from build123d import *

# Parameters (mm, degrees)
F1_DEPTH = 60
F2_R     = 5
F3_SIZE  = 5
F4_R     = 22.693936
F5_DEPTH = 30


with BuildPart() as f1:
    # F0 (on Front) → F1 (new body)
    with BuildSketch(Plane.XZ):
        with BuildLine():
            Line((58.700657, 72.187497), (-16.299343, 72.187497))
            ThreePointArc((-16.299343, 72.187497), (-33.977013, 64.865167), (-41.299343, 47.187497))
            Line((-41.299343, 47.187497), (-41.299343, -27.812503))
            Line((-41.299343, -27.812503), (33.700657, -27.812503))
            ThreePointArc((33.700657, -27.812503), (51.378326, -20.490172), (58.700657, -2.812503))
            Line((58.700657, -2.812503), (58.700657, 72.187497))
        make_face()
    extrude(amount=F1_DEPTH)

    # F2
    f2_edges = [f1.edges().sort_by_distance(p)[0] for p in [
        (58.700657, -60, 34.687497),
        (21.200657, -60, 72.187497),
        (-33.977013, -60, 64.865167),
        (-41.299343, -60, 9.687497),
        (-3.799343, -60, -27.812503),
        (51.378326, -60, -20.490172),
    ]]
    fillet(f2_edges, radius=F2_R)

    # F3
    f3_edges = [f1.edges().sort_by_distance(p)[0] for p in [
        (58.700657, 0, 34.687497),
        (21.200657, 0, 72.187497),
        (-33.977013, 0, 64.865167),
        (-41.299343, 0, 9.687497),
        (-3.799343, 0, -27.812503),
        (51.378326, 0, -20.490172),
    ]]
    chamfer(f3_edges, length=F3_SIZE)

    # F4 (on face) → F5 (cut)
    with BuildSketch(Plane.XZ.offset(60)):
        with Locations((6.069079, 22.94408)):
            Circle(F4_R)
    extrude(amount=-F5_DEPTH, mode=Mode.SUBTRACT)


solid = f1.part
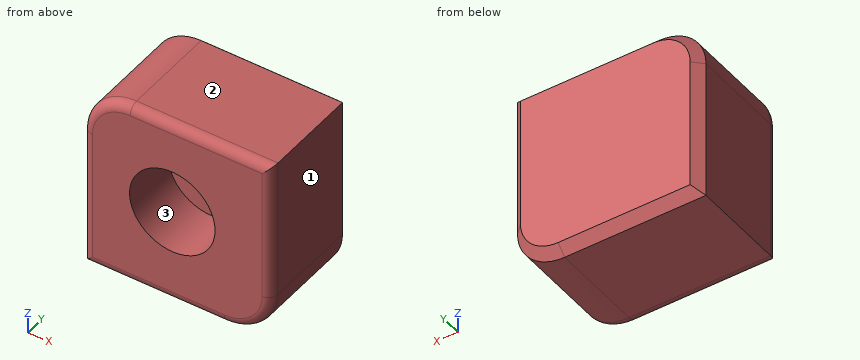
Here's how the part is built. I have some questions about the finished solid (model axes, mm). Face numbers are marked on the shaded views. Coordinates: 2 decimals unless noted, no trailing zeros. Order: outer loops, then holes, each group sorted by start corner. A loop starts at its lowest first (then second) coordinate and runs counter-clockwise, first axis right, second up. Notation, with made-up numbers: (45.5, 63.5) -> (83.5, 63.5) arc R22 cw to (83.5, 73.5) -> close; hole circle Ø2 at (23, 87.25). An arc over 180 degrees is marked (long way). Answer in a Markdown table with one row per item.
(1) Will these pins go through, and if not, where does the flat tip stop? pin 1 Ø22.5 at (x, z) = (-0.5, 12) entering from -Y; pin 2 Ø12 at (x, y) = (42.5, -7) entering from -Z.
Answer key:
| item | result |
|---|---|
| pin 1 | y = -60 |
| pin 2 | z = -27.66 |
(2) Please list where these lines run through material, in increasing order: probe 1 along Y at (x, z) = (-11, 15); probe 2 along X at (y, z) = (-47, 24); probe 3 along Z at (x, y) = (-17.5, -9.5).
Answer key:
| item | result |
|---|---|
| probe 1 | -30 to 0 |
| probe 2 | -41.3 to -16.6, 28.74 to 58.7 |
| probe 3 | -27.81 to 72.16 |
(3) I want a section at A-A on y = -35. List the corners of the cut face in (x, z) for me, then the cut area to 3 significant figures.
Answer key:
| item | result |
|---|---|
| outline | (-41.3, -27.81) -> (33.7, -27.81) arc R25 ccw to (58.7, -2.81) -> (58.7, 72.19) -> (-16.3, 72.19) arc R25 ccw to (-41.3, 47.19) -> close; hole circle Ø45.39 at (6.07, 22.94) |
| area | 8,110 mm^2 |
(4) I want a section at D-D on z = 29. List the corners of the cut face in (x, y) for me.
Answer key:
| item | result |
|---|---|
| outline | (-41.3, -55) arc R5 ccw to (-36.3, -60) -> (-15.8, -60) -> (-15.8, -30) -> (27.94, -30) -> (27.94, -60) -> (53.7, -60) arc R5 ccw to (58.7, -55) -> (58.7, -5) -> (53.7, 0) -> (-36.3, 0) -> (-41.3, -5) -> close |
(5) I want a section at B-B on x = 10. List the corners of the cut face in (y, z) for me, then the cut area to 3 significant figures.
Answer key:
| item | result |
|---|---|
| outline | (-60, -22.81) arc R5 ccw to (-55, -27.81) -> (-5, -27.81) -> (0, -22.81) -> (0, 67.19) -> (-5, 72.19) -> (-55, 72.19) arc R5 ccw to (-60, 67.19) -> (-60, 45.29) -> (-30, 45.29) -> (-30, 0.59) -> (-60, 0.59) -> close |
| area | 4,620 mm^2 |
(6) Thinking about a two-plate mould opening in X: for the marked faces 1, 2 and 3, which applies, +X half, -X half, draft (parallel to the pull), parting line (faces both ways), or undercut?
Answer key:
| item | result |
|---|---|
| face 1 | +X half |
| face 2 | draft |
| face 3 | undercut |
(7) I want a section at C-C on y = -11. List the corners of the cut face in (x, z) for me.
Answer key:
| item | result |
|---|---|
| outline | (-41.3, -27.81) -> (33.7, -27.81) arc R25 ccw to (58.7, -2.81) -> (58.7, 72.19) -> (-16.3, 72.19) arc R25 ccw to (-41.3, 47.19) -> close |
